Part model, mm, in its own coordinate system. Face numbers are marked on the shaded views. A direction names the side the tool comes from. Round coordinates to 2 decimals unless told otherwise and drop trailing zeros. Loops run counter-clockwise (first coordinate to the right, second up) from the corner with the lowest first, then second, coordinate; pieces in that order, holes last.
(1) Probe probe 1 along Y at (x, z) = (-20, 2); probe 2 along Y at (x, z) = (0, 6.5); probe 3 along Y at (x, z) = (0, 4). List the from-to ranges inside material, lowest first.
(2) Cut at C-C on x = 20. List the corners of the cut face in (y, z), then the cut area to 3 significant figures.
(3) Tool access for the marked faces 5, 6 and 7: list every direction of +Z, -Z, +X, -X, +Y, -Y with a clear straight run to the whole face (end or side of a thin tool).
(4) Cut at D-D on z = 2. Count the separate pieces of the cut face and the enclosed holes in it, then the cut area to 3 significant figures.
(5) Cut at A-A on x = 0. List the corners of the cut face in (y, z), then the cut area to 3 significant figures.
(6) Mould opens along X. For the marked faces 1, 2, 3 and 4 say: +X half, -X half, draft (parallel to the pull), parting line (faces both ways), or undercut.
(7) Cut at B-B on y = 0. List the corners of the cut face in (x, z), then the cut area to 3 significant figures.
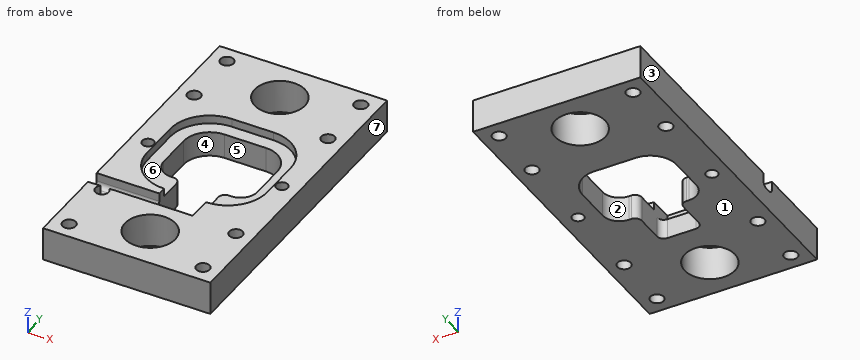
from build123d import *

# Parameters (mm, degrees)
BOSS_EXTRUDE1_DEPTH = 10
CUT_EXTRUDE1_DEPTH  = 11
SKETCH3_W           = 50
SKETCH3_H           = 45
BOSS_EXTRUDE3_DEPTH = 10
CUT_EXTRUDE6_DEPTH  = 2.5
SKETCH5_W           = 12.5
SKETCH5_H           = 6.253832763
CUT_EXTRUDE7_DEPTH  = 4
SKETCH6_W           = 50
SKETCH6_H           = 23.984880812
SKETCH6_R           = 7.5
SKETCH6_H_2         = 25
BOSS_EXTRUDE4_DEPTH = 10
CUT_EXTRUDE8_DEPTH  = 31.25
SKETCH8_R           = 2
SKETCH8_R_2         = 1.75
CUT_EXTRUDE11_DEPTH = 11
SKETCH9_R           = 2
CUT_EXTRUDE12_DEPTH = 11


with BuildPart() as part:
    # Sketch1 → Boss-Extrude1 (new body)
    with BuildSketch(Plane.XY):
        with BuildLine():
            Line((-7, 19), (7, 19))
            ThreePointArc((7, 19), (14.071067812, 16.071067812), (17, 9))
            Line((17, 9), (17, -5))
            ThreePointArc((17, -5), (14.071067812, -12.071067812), (7, -15))
            Line((7, -15), (-7, -15))
            ThreePointArc((-7, -15), (-14.071067812, -12.071067812), (-17, -5))
            Line((-17, -5), (-17, 9))
            ThreePointArc((-17, 9), (-14.071067812, 16.071067812), (-7, 19))
        make_face()
    extrude(amount=BOSS_EXTRUDE1_DEPTH)

    # Sketch2 → Cut-Extrude1 (cut, through all)
    with BuildSketch(Plane(origin=(0, 0, 0), x_dir=(-1, 0, 0), z_dir=(0, 0, -1))):
        with BuildLine():
            Line((14, 0.39), (14, 8.212908396))
            ThreePointArc((14, 8.212908396), (11.719213675, 13.719213675), (6.212908396, 16))
            Line((6.212908396, 16), (-6.212908396, 16))
            ThreePointArc((-6.212908396, 16), (-11.719213675, 13.719213675), (-14, 8.212908396))
            Line((-14, 8.212908396), (-14, 0.39))
            Line((-14, 0.39), (-14, -2.4))
            ThreePointArc((-14, -2.4), (-12.535533906, -5.935533906), (-9, -7.4))
            Line((-9, -7.4), (-8.25, -7.4))
            ThreePointArc((-8.25, -7.4), (-6.835786438, -7.985786438), (-6.25, -9.4))
            Line((-6.25, -9.4), (-6.25, -17.62539529))
            Line((-6.25, -17.62539529), (6.25, -17.62539529))
            Line((6.25, -17.62539529), (6.25, -9.4))
            ThreePointArc((6.25, -9.4), (6.835786438, -7.985786438), (8.25, -7.4))
            Line((8.25, -7.4), (9, -7.4))
            ThreePointArc((9, -7.4), (12.535533906, -5.935533906), (14, -2.4))
            Line((14, -2.4), (14, 0.39))
        make_face()
    extrude(amount=-CUT_EXTRUDE1_DEPTH, mode=Mode.SUBTRACT)

    # Sketch3 → Boss-Extrude3 (add)
    with BuildSketch(Plane(origin=(0, 0, 0), x_dir=(-1, 0, 0), z_dir=(0, 0, -1))):
        with Locations((0, -0.507559594)):
            Rectangle(SKETCH3_W, SKETCH3_H)
        with BuildLine():
            Line((-6.25, -9.4), (-6.25, -15))
            Line((-6.25, -15), (-6.25, -17.5))
            ThreePointArc((-6.25, -17.5), (-5.664213562, -18.914213562), (-4.25, -19.5))
            Line((-4.25, -19.5), (4.25, -19.5))
            ThreePointArc((4.25, -19.5), (5.664213562, -18.914213562), (6.25, -17.5))
            Line((6.25, -17.5), (6.25, -15))
            Line((6.25, -15), (6.25, -9.4))
            ThreePointArc((6.25, -9.4), (6.835786438, -7.985786438), (8.25, -7.4))
            Line((8.25, -7.4), (9, -7.4))
            ThreePointArc((9, -7.4), (12.535533906, -5.935533906), (14, -2.4))
            Line((14, -2.4), (14, 8.212908396))
            ThreePointArc((14, 8.212908396), (11.719213675, 13.719213675), (6.212908396, 16))
            Line((6.212908396, 16), (-6.212908396, 16))
            ThreePointArc((-6.212908396, 16), (-11.719213675, 13.719213675), (-14, 8.212908396))
            Line((-14, 8.212908396), (-14, -2.4))
            ThreePointArc((-14, -2.4), (-12.535533906, -5.935533906), (-9, -7.4))
            Line((-9, -7.4), (-8.25, -7.4))
            ThreePointArc((-8.25, -7.4), (-6.835786438, -7.985786438), (-6.25, -9.4))
        make_face(mode=Mode.SUBTRACT)
    extrude(amount=-BOSS_EXTRUDE3_DEPTH)

    # Sketch4 → Cut-Extrude6 (cut)
    with BuildSketch(Plane.XY.offset(10)):
        with BuildLine():
            Line((-18, 8.192440406), (-18, -4.207559594))
            ThreePointArc((-18, -4.207559594), (-14.543860018, -12.551419612), (-6.2, -16.007559594))
            Line((-6.2, -16.007559594), (6.2, -16.007559594))
            ThreePointArc((6.2, -16.007559594), (14.543860018, -12.551419612), (18, -4.207559594))
            Line((18, -4.207559594), (18, 8.192440406))
            ThreePointArc((18, 8.192440406), (14.543860018, 16.536300424), (6.2, 19.992440406))
            Line((6.2, 19.992440406), (-6.2, 19.992440406))
            ThreePointArc((-6.2, 19.992440406), (-14.543860018, 16.536300424), (-18, 8.192440406))
        make_face()
    extrude(amount=-CUT_EXTRUDE6_DEPTH, mode=Mode.SUBTRACT)

    # Sketch5 → Cut-Extrude7 (cut)
    with BuildSketch(Plane.XY.offset(10)):
        with Locations((0, -19.880643213)):
            Rectangle(SKETCH5_W, SKETCH5_H)
    extrude(amount=-CUT_EXTRUDE7_DEPTH, mode=Mode.SUBTRACT)

    # Sketch6 → Boss-Extrude4 (add)
    with BuildSketch(Plane(origin=(0, 0, 0), x_dir=(-1, 0, 0), z_dir=(0, 0, -1))):
        with Locations((0, -35)):
            Rectangle(SKETCH6_W, SKETCH6_H)
        with Locations((0, -34.492440406)):
            Circle(SKETCH6_R, mode=Mode.SUBTRACT)
        with Locations((0, 34.492440406)):
            Rectangle(SKETCH6_W, SKETCH6_H_2)
        with Locations((0, 34.492440406)):
            Circle(SKETCH6_R, mode=Mode.SUBTRACT)
    extrude(amount=-BOSS_EXTRUDE4_DEPTH)

    # Sketch7 → Cut-Extrude8 (cut)
    with BuildSketch(Plane.ZY.offset(25)):
        with BuildLine():
            Line((10, -18.512440406), (7.5, -18.512440406))
            ThreePointArc((7.5, -18.512440406), (6.439339828, -18.951780234), (6, -20.012440406))
            Line((6, -20.012440406), (6, -21.512440406))
            ThreePointArc((6, -21.512440406), (6.439339828, -22.573100578), (7.5, -23.012440406))
            Line((7.5, -23.012440406), (10, -23.012440406))
            Line((10, -23.012440406), (10, -18.512440406))
        make_face()
    extrude(amount=-CUT_EXTRUDE8_DEPTH, mode=Mode.SUBTRACT)

    # Sketch8 → Cut-Extrude11 (cut, through all)
    with BuildSketch(Plane.XY.offset(10)):
        with Locations((-20, 41.992440406)):
            Circle(SKETCH8_R)
        with Locations((20, 41.992440406)):
            Circle(SKETCH8_R)
        with Locations((-20, 0)):
            Circle(SKETCH8_R_2)
        with Locations((20, 0)):
            Circle(SKETCH8_R_2)
        with Locations((20, -41.992440406)):
            Circle(SKETCH8_R)
        with Locations((-20, -41.992440406)):
            Circle(SKETCH8_R)
    extrude(amount=-CUT_EXTRUDE11_DEPTH, mode=Mode.SUBTRACT)

    # Sketch9 → Cut-Extrude12 (cut, through all)
    with BuildSketch(Plane.XY.offset(10)):
        with Locations((-20, 24.492440406)):
            Circle(SKETCH9_R)
        with Locations((20, 24.492440406)):
            Circle(SKETCH9_R)
        with Locations((20, -24.492440406)):
            Circle(SKETCH9_R)
        with Locations((-20, -24.492440406)):
            Circle(SKETCH9_R)
    extrude(amount=-CUT_EXTRUDE12_DEPTH, mode=Mode.SUBTRACT)


solid = part.part
Final values:
1. probe 1: y = -46.99 to -43.99, -39.99 to -26.49, -22.49 to -1.75, 1.75 to 22.49, 26.49 to 39.99, 43.99 to 46.99
1. probe 2: y = -46.99 to -41.99, -26.99 to -23.01, 16 to 26.99, 41.99 to 46.99
1. probe 3: y = -46.99 to -41.99, -26.99 to -19.5, 16 to 26.99, 41.99 to 46.99
2. outline: (-46.99, 0) - (-43.99, 0) - (-43.99, 10) - (-46.99, 10) - close; (-39.99, 0) - (-26.49, 0) - (-26.49, 10) - (-39.99, 10) - close; (-22.49, 0) - (-1.75, 0) - (-1.75, 10) - (-22.49, 10) - close; (1.75, 0) - (22.49, 0) - (22.49, 10) - (1.75, 10) - close; (26.49, 0) - (39.99, 0) - (39.99, 10) - (26.49, 10) - close; (43.99, 0) - (46.99, 0) - (46.99, 10) - (43.99, 10) - close
2. area: 745 mm2
3. face 5: +Z, -Z
3. face 6: +Z
3. face 7: +Z, -Z, +X, +Y, -Y
4. separate pieces: 1
4. enclosed holes: 13
4. area: 3,460 mm2
5. outline: (-46.99, 0) - (-41.99, 0) - (-41.99, 10) - (-46.99, 10) - close; (-26.99, 0) - (-19.5, 0) - (-19.5, 6) - (-23.01, 6) - (-23.01, 7.38) arc R1.5 cw to (-23.01, 7.5) - (-23.01, 10) - (-26.99, 10) - close; (16, 0) - (26.99, 0) - (26.99, 10) - (19.99, 10) - (19.99, 7.5) - (16, 7.5) - close; (41.99, 0) - (46.99, 0) - (46.99, 10) - (41.99, 10) - close
5. area: 261 mm2
6. face 1: draft
6. face 2: undercut
6. face 3: -X half
6. face 4: undercut
7. outline: (-25, 0) - (-21.75, 0) - (-21.75, 10) - (-25, 10) - close; (-18.25, 0) - (-14, 0) - (-14, 7.5) - (-18, 7.5) - (-18, 10) - (-18.25, 10) - close; (14, 0) - (18.25, 0) - (18.25, 10) - (18, 10) - (18, 7.5) - (14, 7.5) - close; (21.75, 0) - (25, 0) - (25, 10) - (21.75, 10) - close
7. area: 130 mm2
